Work out the finished part from the listing and answer in its coordinate system (mm). Give positions to 0.01 mm unless a question says otherwise; leave off trailing zeros. Order: outer loops, then holes, each group sorted by start corner. A loop starts at its lowest first (then second) coordinate and runs counter-clockwise, first axis right, second up. Notation, with made-up numbers: (55.5, 87.5) - (90.5, 87.5) arc R18 cw to (90.5, 116.5) - close; hole circle Ø9 at (2.5, 60.25). An arc over 180 degrees is marked (long way). Write each question's results on one line, items separated by ' | '.
from build123d import *

# Parameters (mm, degrees)
SKETCH2_W           = 152.4
SKETCH2_H           = 152.4
BOSS_EXTRUDE1_DEPTH = 50.8


with BuildPart() as part:
    # Sketch2 → Boss-Extrude1 (new body)
    with BuildSketch(Plane(origin=(0, 0, 0), x_dir=(1, 0, 0), z_dir=(0, 1, 0))):
        Rectangle(SKETCH2_W, SKETCH2_H)
    extrude(amount=BOSS_EXTRUDE1_DEPTH)

    # Sketch3 → Cut-Revolve1 (revolve, cut)
    with BuildSketch(Plane.XY):
        with BuildLine():
            Line((-19.05, 31.75), (0, 31.75))
            Line((0, 31.75), (0, 50.8))
            Line((0, 50.8), (-38.1, 50.8))
            ThreePointArc((-38.1, 50.8), (-32.520384182, 37.329615818), (-19.05, 31.75))
        make_face()
    revolve(axis=Axis((0, 50.8, 0), (0, -1, 0)), mode=Mode.SUBTRACT)


solid = part.part
1. A cutting plane is placed at A-A, the plane y = 44.5. Write down the section's boundary in (x, z), then the cut area to 3 significant figures.
Answer list:
outline: (-76.2, -76.2) - (76.2, -76.2) - (76.2, 76.2) - (-76.2, 76.2) - close; hole circle Ø74.06 at (0, 0) | area: 18,900 mm^2
2. Straight lines are drawn through the part: line 1 (Z direction, x = 14, y = 39.5); line 2 (Z direction, x = 18, y = 37); line 3 (X direction, y = 35, z = -10.5). For each, find the intervals that lie inside material, in ascending order. Write a range as [from, to].
Answer list:
line 1: [-76.2, -31.41], [31.41, 76.2] | line 2: [-76.2, -26.68], [26.68, 76.2] | line 3: [-76.2, -27.77], [27.77, 76.2]
3. Given P1, Ø4, axis at x = 21, z = -26, coming from the +Y side; P2, Ø10, axis at x = 3, z = 14.5, coming from the +Y side, each flat-ended and moving along its own axis, determine where each tip first touches the part or whether it passes through.
Answer list:
P1: y = 41.06 | P2: y = 31.77
4. Determine the mould class of faces 1 (the face through (-76.2, 25, 1)), 2 (the face through (76.2, 25, 1)), 3 (the face through (-1, 0, -1)), 4 (the face through (0, 31.75, 0)) for opening direction X: +X half, -X half, draft (parallel to the pull), parting line (faces both ways), or undercut.
Answer list:
face 1: -X half | face 2: +X half | face 3: draft | face 4: undercut
